```python
from build123d import *

# Parameters (mm, degrees)
BOSS_EXTRUDE1_DEPTH     = 300
FILLET1_R               = 40
CHAMFER1_SIZE           = 10
CHAMFER1_SIZE2          = 2.679491924
CUT_EXTRUDE1_DEPTH      = 336.036145422
CUT_EXTRUDE1_DEPTH_BACK = 336.036145422
SKETCH4_W               = 79.364416539
SKETCH4_H               = 3
BOSS_EXTRUDE2_DEPTH     = 10
SKETCH5_R               = 5.704192845
SKETCH5_R_2             = 4
BOSS_EXTRUDE3_DEPTH     = 80
SKETCH7_R               = 4
CUT_EXTRUDE2_DEPTH      = 80


with BuildPart() as part:
    # Sketch1 → Boss-Extrude1 (new body)
    with BuildSketch(Plane(origin=(0, 0, 0), x_dir=(0, 0, -1), z_dir=(1, 0, 0))):
        Polygon((84.922374429, -7.245973585), (84.922374429, -55.316210046), (7.922374429, -55.316210046), (7.922374429, -58.316210046), (87.922374429, -58.316210046), (87.922374429, -8.272692249), (106.273520759, 15.397445577), (137.289614993, 15.397445577), (137.289614993, 18.397445577), (104.803379808, 18.397445577), align=None)
    extrude(amount=BOSS_EXTRUDE1_DEPTH)

    # Fillet1
    fillet1_edges = [part.edges().sort_by_distance(p)[0] for p in [
        (150, -55.316210046, -84.922374429),
    ]]
    fillet(fillet1_edges, radius=FILLET1_R)

    # Chamfer1
    chamfer1_edges = [part.edges().sort_by_distance(p)[0] for p in [
        (150, -55.316210046, -7.922374429),
    ]]
    chamfer1_side = [part.faces().sort_by_distance(p)[0] for p in [
        (150, -55.316210046, -26.422374429),
    ]]
    chamfer(chamfer1_edges, length=CHAMFER1_SIZE, length2=CHAMFER1_SIZE2, reference=chamfer1_side[0])

    # Sketch2 → Cut-Extrude1 (cut, two sides: drawn at the far end of the back side and taken through both)
    with BuildSketch(Plane(origin=(0, 0, 0), x_dir=(1, 0, 0), z_dir=(0, 1, 0)).offset(-CUT_EXTRUDE1_DEPTH_BACK)):
        Polygon((229.364416539, 137.289614993), (300, 104.803379808), (319.87920565, 121.046497401), (319.87920565, 155.206469458), (246.417927531, 173.123323923), align=None)
        Polygon((150, 137.289614993), (0, 104.803379808), (-27.422104743, 146.559201032), (121.140212168, 173.123323923), align=None)
    extrude(amount=CUT_EXTRUDE1_DEPTH + CUT_EXTRUDE1_DEPTH_BACK, mode=Mode.SUBTRACT)

    # Sketch4 → Boss-Extrude2 (add)
    with BuildSketch(Plane(origin=(0, 0, -137.289614993), x_dir=(-1, 0, 0), z_dir=(0, 0, -1))):
        with Locations((-189.682208269, 16.897445577)):
            Rectangle(SKETCH4_W, SKETCH4_H)
    extrude(amount=BOSS_EXTRUDE2_DEPTH)

    # Sketch5 → Boss-Extrude3 (add)
    with BuildSketch(Plane(origin=(229.364416539, 0, 0), x_dir=(0, 0, -1), z_dir=(1, 0, 0))):
        with Locations((142.289614993, 16.897445577)):
            Circle(SKETCH5_R)
        with Locations((142.289614993, 16.897445577)):
            Circle(SKETCH5_R_2, mode=Mode.SUBTRACT)
    extrude(amount=-BOSS_EXTRUDE3_DEPTH)

    # Sketch7 → Cut-Extrude2 (cut)
    with BuildSketch(Plane(origin=(229.364416539, 0, 0), x_dir=(0, 0, -1), z_dir=(1, 0, 0))):
        with Locations((142.289614993, 16.897445577)):
            Circle(SKETCH7_R)
    extrude(amount=-CUT_EXTRUDE2_DEPTH, mode=Mode.SUBTRACT)


solid = part.part
```
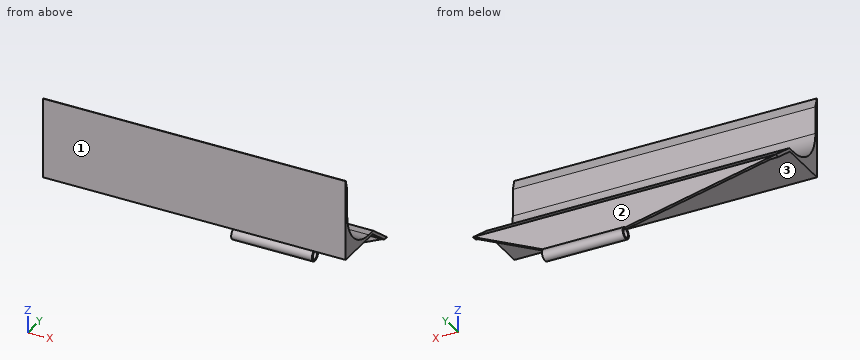
Work out the finished part from the listing and answer in its coordinate system (mm). Face numbers are marked on the shaded views. A direction names the side the tool comes from. Round coordinates to 2 decimals unless told otherwise and drop trailing zeros. Write each loop counter-clockwise with the first axis right and the second up, starting at its lowest first coordinate (ties: lowest second). Pieces come first, ordered by that corner, then holes.
1) Which of the six approach directions +Z, -Z, +X, -X, +Y, -Y give full straight-line access (tool end or side, diameter ignored) to the marked faces 1, 2 and 3?
2) Flat-ended cylindrical pins translate along their axes: P1, Ø12, axis at x = 131.5, z = -130.5, coming from the +Y side; P2, Ø6, axis at x = 123.5, y = -30.5, coming from the -Z side; P3, Ø9, axis at y = 15.5, z = -142, coming from the -X side; P4, Ø10, axis at y = -0.5, z = -85.5, coming from the -X side. Find the tip coordinate at first contact, or state that the pin passes through.
3) A cutting plane is placed at B-B on z = -40. Determine the outline of the cut face in (x, y).
4) Consider probe 1 along Y at (x, z) = (235, -34.5); probe 2 along Z at (x, y) = (202.5, -10); probe 3 along Y at (x, z) = (260.5, -110). Determine where each line is inside the solid, lowest interval first.
5) A cutting plane is placed at D-D on y = -45. Determine the outline of the cut face in (x, z).
6) A cutting plane is placed at C-C on x = 206. Determine the outline of the cut face in (y, z).
7) A cutting plane is placed at A-A on x = 112. Determine the outline of the cut face in (y, z).
Entries:
1. face 1: +Z, -Z, +X, -X, -Y
1. face 2: +Z, +X, -X, +Y
1. face 3: -Z, +X, -X, -Y
2. P1: stops at y = 18.4
2. P2: stops at z = -87.92
2. P3: stops at x = 149.36
2. P4: stops at x = 0
3. outline: (0, -58.32) - (300, -58.32) - (300, -55.32) - (0, -55.32) - close
4. probe 1: y = -58.32 to -55.32
4. probe 2: z = -87.92 to -84.92
4. probe 3: y = 15.4 to 18.4
5. outline: (0, -87.92) - (300, -87.92) - (300, -71.73) - (0, -71.73) - close
6. outline: (-58.32, -87.92) - (-8.27, -87.92) - (15.4, -106.27) - (15.4, -136.79) arc R5.7 ccw (long way) to (18.4, -136.79) - (18.4, -104.8) - (-7.25, -84.92) - (-15.32, -84.92) arc R40 cw to (-55.32, -44.92) - (-55.32, -17.92) - (-58, -7.92) - (-58.32, -7.92) - close; hole circle Ø8 at (16.9, -142.29)
7. outline: (-58.32, -87.92) - (-8.27, -87.92) - (15.4, -106.27) - (15.4, -129.06) - (18.4, -129.06) - (18.4, -104.8) - (-7.25, -84.92) - (-15.32, -84.92) arc R40 cw to (-55.32, -44.92) - (-55.32, -17.92) - (-58, -7.92) - (-58.32, -7.92) - close
